Autodesk Inventor part; units mm, degrees
ref_plane "YZ Plane" through (0, 0, 0) normal (1, 0, 0) x (0, 1, 0)
ref_plane "XZ Plane" through (0, 0, 0) normal (0, 1, 0) x (-1, 0, 0)
ref_plane "XY Plane" through (0, 0, 0) normal (0, 0, 1) x (1, 0, 0)
sketch "Skizze1" plane through (0, 0, 0) normal (0, 0, 1) x (1, 0, 0)
  line L0 (0, 0) -> (1.7032, 0)
  line L1 (2, 2) -> (2, 30)
  line L2 (2, 30) -> (0, 30)
  line L3 (0, 30) -> (0, 0)
  line L4 (0, 0) -> (15, 0)
  line L5 (15, 0) -> (15, 2)
  line L6 (15, 2) -> (2, 2)
  line L7 (0, 2.129) -> (0, 0)
  dimension "d0" = 30
  dimension "d1" = 15
  dimension "d2" = 2
extrude "Extrusion1" add sketch "Skizze1" along normal blind 15
sketch "Skizze2" plane through (0, 0, 0) normal (-1, 0, 0) x (0, 0, 1)
  line L0 (0, 30) -> (15, 30)
  line L1 (0, 0) -> (0, 30)
  line L2 (0, 0) -> (15, 0)
  line L3 (0, -6) -> (0, 36)
  line L4 (-3, 0) -> (18, 0)
  line L5 (7.5, 30) -> (7.5, 0)
  point P0 (7.5, 15)
  dimension "d5" = 30
  dimension "d6" = 7.5
  dimension "d7" = 15
hole "Bohrung1" at (0, 15, 7.5) direction (1, 0, 0) diameter 6 end through all
sketch "Skizze3" plane through (2, 2, 0) normal (0, 1, 0) x (1, 0, 0)
  line L0 (0, -15) -> (13, -15)
  line L1 (0, 0) -> (0, -15)
  line L2 (13, 0) -> (0, 0)
  line L3 (0, 0) -> (0, -7)
  line L4 (0, -7) -> (13, -7)
  line L5 (13, -7) -> (13, 0)
  point P0 (-2, 0)
  dimension "d15" = 8
extrude "Extrusion2" cut sketch "Skizze3" against normal through all
sketch "Skizze4" plane through (2, 0, 0) normal (1, 0, 0) x (0, 0, -1)
  line L0 (-15, 30) -> (-15, 2)
  line L1 (0, 30) -> (0, 0)
  line L2 (0, 30) -> (-15, 30)
  line L3 (-15, 27.5) -> (0, 27.5)
  line L4 (-15, 22) -> (0, 22)
  point P0 (-11, 25)
  point P1 (-4, 25)
  dimension "d18" = 2.5
  dimension "d19" = 8
  dimension "d20" = 5
  dimension "d21" = 5
  dimension "d22" = 4
  dimension "d23" = 4
hole "Bohrung2" at (2, 25, 11) at (2, 25, 4) direction (-1, 0, 0) diameter 3.4 end through all
sketch "Skizze5" plane through (2, 2, 15) normal (0, 1, 0) x (1, 0, 0)
  line L0 (13, 8) -> (0, 8)
  line L1 (13, 8) -> (13, 0)
  point P0 (-2, 15)
  point P1 (5.5, 4)
  dimension "d31" = 7.5
  dimension "d32" = 4
hole "Bohrung3" at (7.5, 2, 11) direction (0, -1, 0) diameter 4.5 end through all
hole "Bohrung4" at (2, 25, 4) direction (-1, 0, 0) diameter 3.4 end through all countersink diameter 6 countersink angle 90
chamfer "Fase1" distance 2 angle 45 2 edges at (15, 1, 15) (15, 1, 7)
properties part number "13_0204_051"
Part model, mm, in its own coordinate system. A direction names the side the tool comes from. Round coordinates to 2 decimals unless told otherwise and drop trailing zeros. Write each loop counter-clockwise with the first axis right and the second up, starting at its lowest first coordinate (ties: lowest second). Pieces come first, ordered by that corner, then holes. Notation, with made-up numbers: M -33,77 L 17,77 A4 cw 17,81 Z; hole C -3,79.5 d1. An arc over 180 degrees is marked long. Answer as CSV lines item,"result". Start each with the question number.
1) Band-saw the part on C-C (y = 15). List the corners of the cut face in (x, z).
2) Band-saw the part on D-D (z = 8.25). List the corners of the cut face in (x, y), then the cut area to 3 significant figures.
3) Drill centre lines: L1, parallel to Y at x = 1, z = 7.5; L2, parallel to Y at x = 0.5, z = 4; L3, parallel to Z at x = 0.4, y = 25. Where is each one in solid material? Low to high.
4) Band-saw the part on B-B (y = 25). List the corners of the cut face in (x, z).
5) Band-saw the part on A-A (x = 7.5). List the corners of the cut face in (y, z), then the cut area to 3 significant figures.
6) Mould opens along Z. For faces 3 (the face through (0.986, 23.567, 10.086)), 4 (the face through (1, 27, 4)), 5 (the face through (10, 2, 11)), 6 (the face through (1, 15, 0)) say: +Z half, -Z half, draft (parallel to the pull), parting line (faces both ways), or undercut.
7) Which spindle directions (+Z, -Z, +X, -X, +Y, -Y) get a long thin tool onto all of the face, cutting with end or side? Do faces 1 (the face through (7, 1, 7)), 2 (the face through (14, 1, 14)). Say none if no direction does.
8) Drop flat-ended pins along their axis: pin 1 (4 mm diameter, centred on x = 7.5, z = 10, fed in from +Y); pin 2 (6 mm diameter, centred on x = 7.5, z = 11, fed in from -Y); pin 3 (1 mm diameter, centred on x = 10, y = 0.5, fed in from -Z); pin 4 (5.5 mm diameter, centred on y = 25, z = 11, fed in from +X). Give the stop position or say it passes through.
Worked out:
1,outline,"M 0,0 L 2,0 L 2,4.5 L 0,4.5 Z; M 0,10.5 L 2,10.5 L 2,15 L 0,15 Z"
2,outline,"M 0,0 L 14.25,0 L 14.25,2 L 2,2 L 2,12.1 L 0,12.1 Z; M 0,17.9 L 2,17.9 L 2,30 L 0,30 Z"
2,area,"72.9 mm²"
3,L1,"0 to 12, 18 to 30"
3,L2,"0 to 23.3, 26.7 to 30"
3,L3,"0 to 2.3, 5.7 to 9.3, 12.7 to 15"
4,outline,"M 0,0 L 2,0 L 2,1 L 0.7,2.3 L 0,2.3 Z; M 0,5.7 L 0.7,5.7 L 2,7 L 2,9.3 L 0,9.3 Z; M 0,12.7 L 2,12.7 L 2,15 L 0,15 Z"
5,outline,"M 0,7 L 2,7 L 2,8.75 L 0,8.75 Z; M 0,13.25 L 2,13.25 L 2,15 L 0,15 Z"
5,area,"7.00 mm²"
6,face 3,"undercut"
6,face 4,"undercut"
6,face 5,"draft"
6,face 6,"-Z half"
7,face 1,"-Z, +X, +Y, -Y"
7,face 2,"+Z, +X, +Y, -Y"
8,pin 1,"y = 2"
8,pin 2,"y = 0"
8,pin 3,"z = 7"
8,pin 4,"x = 2"
